Part print with two shaded views. Sizes in mm from the minimum x, y, z corner. Round coordinates to 2 decimals unless told otherwise and drop trailing zeros. Order: outer loops, then holes, each group sorted by start corner. A loop starts at its lowest first (then second) coordinate and runs counter-clockwise, first axis right, second up. Notation, with made-up numbers: (15, -32) - (74, -32) arc R14 ccw to (74, -7) - close; hole circle Ø1 at (81, -25). An arc over 180 degrees is marked (long way). Use one line per item in the form item = value.
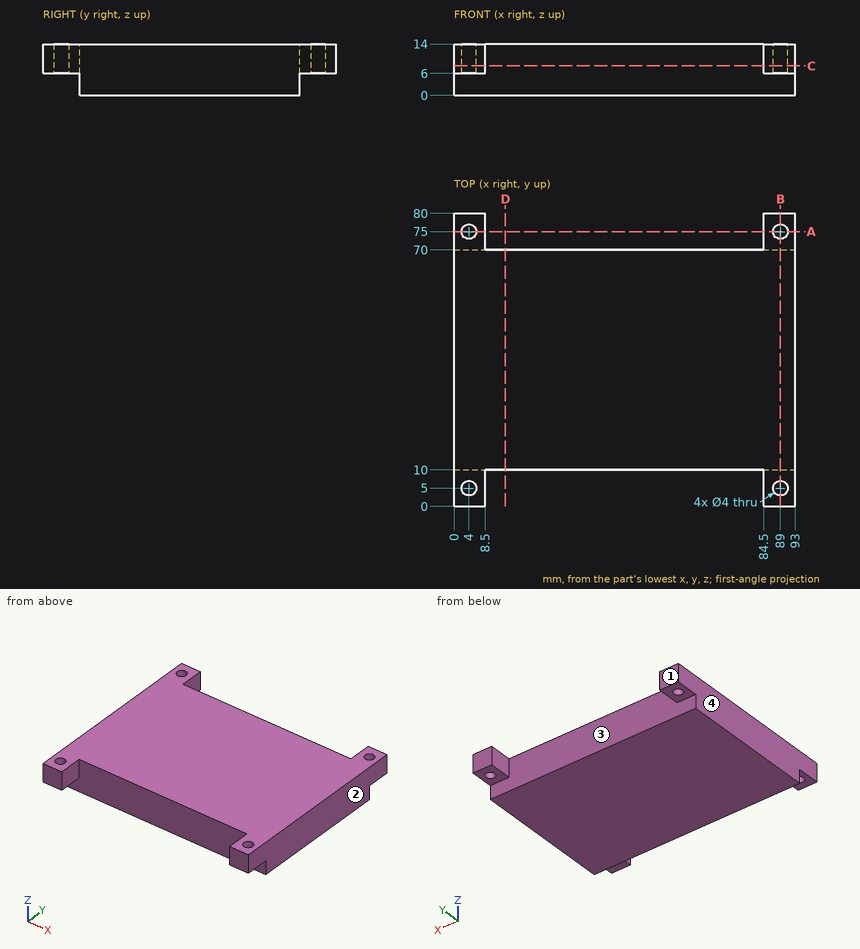
(1) Probe probe 1 along Y at (x, z) = (4, 12.25); probe 2 along X at (y, z) = (75, 10.25); probe 3 along Y at (x, z) = (60.5, 13). List the from-to ranges inside material, lowest first. Write a range as [from, to].
Report:
probe_1 = [0, 3], [7, 73], [77, 80]
probe_2 = [0, 2], [6, 8.5], [84.5, 87], [91, 93]
probe_3 = [10, 70]
(2) Slice it at B-B on x = 89. Give the cut face in (y, z).
Report:
outline = (0, 6) - (3, 6) - (3, 14) - (0, 14) - close; (7, 6) - (10, 6) - (10, 0) - (70, 0) - (70, 6) - (73, 6) - (73, 14) - (7, 14) - close; (77, 6) - (80, 6) - (80, 14) - (77, 14) - close
(3) Pin check, flat tips, straight feed: pin 1 (2.5 mm diameter, centred on x = 4, y = 3, fed in from -Z); pin 2 (4 mm diameter, centred on x = 34, z = 4, fed in from -Y). Stop position of each tip, or through.
Report:
pin_1 = 6
pin_2 = 10
(4) Slice it at A-A on y = 75. Give the cut face in (x, z), then the cut area to 3 significant figures.
Report:
outline = (0, 6) - (2, 6) - (2, 14) - (0, 14) - close; (6, 6) - (8.5, 6) - (8.5, 14) - (6, 14) - close; (84.5, 6) - (87, 6) - (87, 14) - (84.5, 14) - close; (91, 6) - (93, 6) - (93, 14) - (91, 14) - close
area = 72.0 mm2
(5) Pull direction X, two halves, no side cores. Call the marked faces 1, 2, 3 and 4: released by +X, released by -X, zero draft, split by the parting line, or undercut.
Report:
face_1 = zero draft
face_2 = released by +X
face_3 = undercut
face_4 = released by -X
(6) Slice it at D-D on x = 14. Give the cut face in (y, z).
Report:
outline = (10, 0) - (70, 0) - (70, 14) - (10, 14) - close
(7) Slice it at C-C on z = 8. Give the cut face in (x, y).
Report:
outline = (0, 0) - (8.5, 0) - (8.5, 10) - (84.5, 10) - (84.5, 0) - (93, 0) - (93, 80) - (84.5, 80) - (84.5, 70) - (8.5, 70) - (8.5, 80) - (0, 80) - close; hole circle Ø4 at (4, 5); hole circle Ø4 at (4, 75); hole circle Ø4 at (89, 5); hole circle Ø4 at (89, 75)
